```python
from build123d import *

# Parameters (mm, degrees)
SKETCH1_R           = 0.95
SKETCH1_R_2         = 2.949148862
BOSS_EXTRUDE1_DEPTH = 5
SKETCH2_R           = 2
CUT_EXTRUDE1_DEPTH  = 2
BOSS_EXTRUDE2_START = -7
SKETCH1_3_R         = 18.5
BOSS_EXTRUDE2_DEPTH = 7


with BuildPart() as part:
    # Sketch1 → Boss-Extrude1 (new body)
    with BuildSketch(Plane.XY):
        with BuildLine():
            Line((20.851596989, 10.883974596), (19.851596989, 12.616025404))
            Line((19.851596989, 12.616025404), (17.232385626, 11.103823019))
            ThreePointArc((17.232385626, 11.103823019), (10.25, 17.753520778), (1, 20.475595229))
            Line((1, 20.475595229), (1, 23.5))
            Line((1, 23.5), (-1, 23.5))
            Line((-1, 23.5), (-1, 20.475595229))
            ThreePointArc((-1, 20.475595229), (-10.25, 17.753520778), (-17.232385626, 11.103823019))
            Line((-17.232385626, 11.103823019), (-19.851596989, 12.616025404))
            Line((-19.851596989, 12.616025404), (-20.851596989, 10.883974596))
            Line((-20.851596989, 10.883974596), (-18.232385626, 9.371772211))
            ThreePointArc((-18.232385626, 9.371772211), (-20.5, 0), (-18.232385626, -9.371772211))
            Line((-18.232385626, -9.371772211), (-20.851596989, -10.883974596))
            Line((-20.851596989, -10.883974596), (-19.851596989, -12.616025404))
            Line((-19.851596989, -12.616025404), (-17.232385626, -11.103823019))
            ThreePointArc((-17.232385626, -11.103823019), (-10.25, -17.753520778), (-1, -20.475595229))
            Line((-1, -20.475595229), (-1, -23.5))
            Line((-1, -23.5), (1, -23.5))
            Line((1, -23.5), (1, -20.475595229))
            ThreePointArc((1, -20.475595229), (10.25, -17.753520778), (17.232385626, -11.103823019))
            Line((17.232385626, -11.103823019), (19.851596989, -12.616025404))
            Line((19.851596989, -12.616025404), (20.851596989, -10.883974596))
            Line((20.851596989, -10.883974596), (18.232385626, -9.371772211))
            ThreePointArc((18.232385626, -9.371772211), (20.5, 0), (18.232385626, 9.371772211))
            Line((18.232385626, 9.371772211), (20.851596989, 10.883974596))
        make_face()
        with Locations((10.5, 0)):
            Circle(SKETCH1_R, mode=Mode.SUBTRACT)
        with Locations((-5.25, -9.09)):
            Circle(SKETCH1_R, mode=Mode.SUBTRACT)
        with Locations((-5.25, 9.09)):
            Circle(SKETCH1_R, mode=Mode.SUBTRACT)
        Circle(SKETCH1_R_2, mode=Mode.SUBTRACT)
    extrude(amount=BOSS_EXTRUDE1_DEPTH)

    # Sketch2 → Cut-Extrude1 (cut)
    with BuildSketch(Plane.XY.offset(5)):
        with Locations((-5.25, 9.09)):
            Circle(SKETCH2_R)
        with Locations((-5.25, -9.09)):
            Circle(SKETCH2_R)
        with Locations((10.5, 0)):
            Circle(SKETCH2_R)
    extrude(amount=-CUT_EXTRUDE1_DEPTH, mode=Mode.SUBTRACT)

    # Sketch1<3> → Boss-Extrude2 (add)
    with BuildSketch(Plane.XY.offset(BOSS_EXTRUDE2_START)):
        with BuildLine():
            Line((20.851596989, 10.883974596), (19.851596989, 12.616025404))
            Line((19.851596989, 12.616025404), (17.232385626, 11.103823019))
            ThreePointArc((17.232385626, 11.103823019), (10.25, 17.753520778), (1, 20.475595229))
            Line((1, 20.475595229), (1, 23.5))
            Line((1, 23.5), (-1, 23.5))
            Line((-1, 23.5), (-1, 20.475595229))
            ThreePointArc((-1, 20.475595229), (-10.25, 17.753520778), (-17.232385626, 11.103823019))
            Line((-17.232385626, 11.103823019), (-19.851596989, 12.616025404))
            Line((-19.851596989, 12.616025404), (-20.851596989, 10.883974596))
            Line((-20.851596989, 10.883974596), (-18.232385626, 9.371772211))
            ThreePointArc((-18.232385626, 9.371772211), (-20.5, 0), (-18.232385626, -9.371772211))
            Line((-18.232385626, -9.371772211), (-20.851596989, -10.883974596))
            Line((-20.851596989, -10.883974596), (-19.851596989, -12.616025404))
            Line((-19.851596989, -12.616025404), (-17.232385626, -11.103823019))
            ThreePointArc((-17.232385626, -11.103823019), (-10.25, -17.753520778), (-1, -20.475595229))
            Line((-1, -20.475595229), (-1, -23.5))
            Line((-1, -23.5), (1, -23.5))
            Line((1, -23.5), (1, -20.475595229))
            ThreePointArc((1, -20.475595229), (10.25, -17.753520778), (17.232385626, -11.103823019))
            Line((17.232385626, -11.103823019), (19.851596989, -12.616025404))
            Line((19.851596989, -12.616025404), (20.851596989, -10.883974596))
            Line((20.851596989, -10.883974596), (18.232385626, -9.371772211))
            ThreePointArc((18.232385626, -9.371772211), (20.5, 0), (18.232385626, 9.371772211))
            Line((18.232385626, 9.371772211), (20.851596989, 10.883974596))
        make_face()
        Circle(SKETCH1_3_R, mode=Mode.SUBTRACT)
    extrude(amount=BOSS_EXTRUDE2_DEPTH)


solid = part.part
```
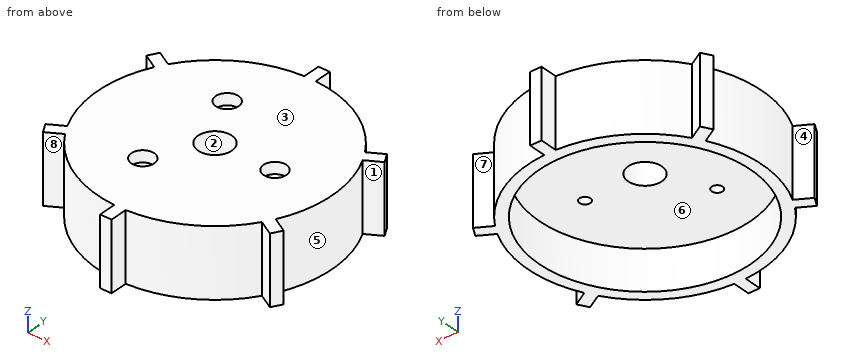
The model under review builds one solid part; all positions refer to its coordinate system, in mm. Face numbers are marked on the shaded views. A direction names the side the tool comes from. Give positions to 0.01 mm unless a question says otherwise; leave off trailing zeros. Write each loop counter-clockwise with the first axis right and the second up, starting at its lowest first coordinate (ties: lowest second). Pieces come first, ordered by that corner, then holes. Notation, with made-up numbers: M 66,46.25 L 100,46.25 A22 cw 100,52.25 Z; hole C 17.25,66.25 d5. An arc over 180 degrees is marked long. Write each question's results on one line, items separated by ' | '. Start each with the question number.
1. Mouldability with a two-part tool opening along X and no side actions: class the marked faces 1, 2, 3 and 4 as released by +X, released by -X, zero draft, split by the parting line, or undercut.
2. For probe 1 along Y at (x, z) = (-5.25, 3.9); probe 2 along X at (y, z) = (12, -6.5); probe 3 along X at (y, z) = (-12.5, 4.5), list the stretches that pass through material, from the lowest coordinate up. Write a range as [from, to].
3. We need section A-A (y = 0). Write out the cut boundary in (x, z).
4. We need section C-C (z = 1.5). Write out the cut boundary in (x, y).
5. Insertion check: pin 1 Ø1.5 at (y, z) = (-21.5, -3) entering from -X; pin 2 Ø4 at (x, z) = (-6.5, -4) entering from -Y; pin 3 Ø4 at (y, z) = (-15, 1.5) entering from +X. Each pin has a flat end and moves straight along its axis. Give the tip position at first contact, or say it passes through.
6. We need section D-D (x = -5). Write out the cut boundary in (y, z).
7. For the marked faces 5, 6, 7 and 8, list the 3-axis set-ups (+Z, -Z, +X, -X, +Y, -Y) from which the entire face can be reached by the end or side of a thin tool; tool diameter is ignored.
8. We need section B-B (x = 0). Write out the cut boundary in (y, z).
Results found:
1) face 1: released by +X | face 2: undercut | face 3: zero draft | face 4: released by -X
2) probe 1: y = [-19.82, -11.09], [-7.09, 7.09], [11.09, 19.82] | probe 2: x = [-20.21, -18.78], [-16.62, -14.08], [14.08, 16.62], [18.78, 20.21] | probe 3: x = [-19.92, -19.65], [-16.25, 16.25], [19.65, 19.92]
3) outline: M -20.5,-7 L -18.5,-7 L -18.5,0 L -2.95,0 L -2.95,5 L -20.5,5 Z; M 2.95,0 L 9.55,0 L 9.55,3 L 8.5,3 L 8.5,5 L 2.95,5 Z; M 11.45,0 L 18.5,0 L 18.5,-7 L 20.5,-7 L 20.5,5 L 12.5,5 L 12.5,3 L 11.45,3 Z
4) outline: M -20.85,-10.88 L -19.85,-12.62 L -17.23,-11.1 A20.5 ccw -1,-20.48 L -1,-23.5 L 1,-23.5 L 1,-20.48 A20.5 ccw 17.23,-11.1 L 19.85,-12.62 L 20.85,-10.88 L 18.23,-9.37 A20.5 ccw 18.23,9.37 L 20.85,10.88 L 19.85,12.62 L 17.23,11.1 A20.5 ccw 1,20.48 L 1,23.5 L -1,23.5 L -1,20.48 A20.5 ccw -17.23,11.1 L -19.85,12.62 L -20.85,10.88 L -18.23,9.37 A20.5 ccw -18.23,-9.37 Z; hole C -5.25,-9.09 d1.9; hole C -5.25,9.09 d1.9; hole C 0,0 d5.9; hole C 10.5,0 d1.9
5) pin 1: stops at x = -1 | pin 2: stops at y = -20 | pin 3: stops at x = 15.85
6) outline: M -19.88,-7 L -17.81,-7 L -17.81,0 L -10.01,0 L -10.01,3 L -11.07,3 L -11.07,5 L -19.88,5 Z; M -8.17,0 L 8.17,0 L 8.17,3 L 7.11,3 L 7.11,5 L -7.11,5 L -7.11,3 L -8.17,3 Z; M 10.01,0 L 17.81,0 L 17.81,-7 L 19.88,-7 L 19.88,5 L 11.07,5 L 11.07,3 L 10.01,3 Z
7) face 5: +Z, -Z, +X | face 6: -Z | face 7: +Z, -Z, +Y | face 8: +Z, -Z, -Y
8) outline: M -23.5,-7 L -18.5,-7 L -18.5,0 L -2.95,0 L -2.95,5 L -23.5,5 Z; M 2.95,0 L 18.5,0 L 18.5,-7 L 23.5,-7 L 23.5,5 L 2.95,5 Z
